Autodesk Inventor part; units mm, degrees
ref_plane "YZ Plane" through (0, 0, 0) normal (1, 0, 0) x (0, 1, 0)
ref_plane "XZ Plane" through (0, 0, 0) normal (0, 1, 0) x (-1, 0, 0)
ref_plane "XY Plane" through (0, 0, 0) normal (0, 0, 1) x (1, 0, 0)
sketch "Sketch1" plane through (0, 0, 0) normal (0, 0, 1) x (1, 0, 0)
  line L0 (-41, -50) -> (41, -50)
  line L1 (41, -50) -> (41, 50)
  line L2 (41, 50) -> (-41, 50)
  line L3 (-41, 50) -> (-41, -50)
  line L4 (-41, -50) -> (41, 50) construction
  line L5 (41, -50) -> (-41, 50) construction
  point P0 (0, 0)
  dimension "d154" = 82
  dimension "d155" = 100
extrude "Plate5" add sketch "Sketch1" along normal blind 2
sketch "Sketch7" plane through (-39, -50, 0) normal (-1, 0, 0) x (0, -1, 0)
  line L0 (-100, 0) -> (0, 0)
  line L1 (0, 0) -> (0, 84)
  line L2 (0, 84) -> (-100, 84)
  line L3 (-100, 84) -> (-100, 0)
edge flange "Flange3" height 84 angle 90 thickness 2 bend radius 2.75 thickness toward (-1, 0, 0) relief round relief width 2 relief depth 1 edges at (-41, 0, 2) wall of the first edge with corners at (-39, 50, 0) (-39, -50, 0) (-39, -50, 84) (-39, 50, 84)
bend "Bend3"
corner "Corner3"
sketch "Sketch8" plane through (0, 0, 2) normal (0, 0, 1) x (1, 0, 0)
  line L0 (41, 50) -> (41, -50)
  line L1 (-36.25, 50) -> (41, 50)
  line L2 (30.375, 42) -> (-25.625, 42)
  line L3 (-25.625, 42) -> (-25.625, -14)
  line L4 (-25.625, -14) -> (30.375, -14)
  line L5 (30.375, -14) -> (30.375, 42)
  line L6 (30.375, 42) -> (-25.625, -14) construction
  line L7 (-25.625, 42) -> (30.375, -14) construction
  point P0 (0, 0)
  point P1 (2.375, 14)
  point P2 (2.375, 50)
  dimension "d167" = 56
  dimension "d168" = 56
  dimension "d169" = 8
extrude "Cut1" cut sketch "Sketch8" against normal blind 2
sketch "Sketch9" plane through (-41, -50, 84) normal (-1, 0, 0) x (0, 0, 1)
  line L0 (-24.375, 44.75) -> (-54.875, 44.75)
  line L1 (-54.875, 44.75) -> (-54.875, 75.25)
  line L2 (-54.875, 75.25) -> (-24.375, 75.25)
  line L3 (-24.375, 75.25) -> (-24.375, 44.75)
  line L4 (-24.375, 44.75) -> (-54.875, 75.25) construction
  line L5 (-54.875, 44.75) -> (-24.375, 75.25) construction
  circle A0 centre (-16.625, 37) radius 2.5
  circle A1 centre (-62.625, 37) radius 2.5
  circle A2 centre (-62.625, 83) radius 2.5
  circle A3 centre (-16.625, 83) radius 2.5
  circle A4 centre (-39.625, 60) radius 32.5269 construction
  line L6 (-54.875, 44.75) -> (-62.625, 37) construction
  line L7 (-14.125, 34.5) -> (-65.125, 34.5) construction
  line L8 (-65.125, 34.5) -> (-65.125, 85.5) construction
  line L9 (-65.125, 85.5) -> (-14.125, 85.5) construction
  line L10 (-14.125, 85.5) -> (-14.125, 34.5) construction
  line L11 (-14.125, 34.5) -> (-65.125, 85.5) construction
  line L12 (-65.125, 34.5) -> (-14.125, 85.5) construction
  line L13 (-79.25, 100) -> (0, 100)
  line L14 (-39.625, 100) -> (-39.625, 60) construction
  circle A5 centre (-62.625, 83) radius 10.9602 construction
  line L15 (-16.625, 37) -> (-62.625, 37) construction
  line L16 (-62.625, 37) -> (-62.625, 83) construction
  line L17 (-62.625, 83) -> (-16.625, 83) construction
  line L18 (-16.625, 83) -> (-16.625, 37) construction
  line L19 (-16.625, 37) -> (-62.625, 83) construction
  line L20 (-62.625, 37) -> (-16.625, 83) construction
  point P0 (-84, 50)
  point P1 (-104.8197, 150.8767)
  point P2 (-104.8197, 150.8767)
  dimension "d181" = 21.9203
  dimension "d174" = 30.5
  dimension "d175" = 30.5
  dimension "d176" = 5
  dimension "d179" = 40
  dimension "d180" = 51
  dimension "d184" = 46
extrude "Cut2" cut sketch "Sketch9" against normal blind 2
properties part number "PRS 940-510 FDS Central tube wall" material "Stainless Steel"
Part model, mm, in its own coordinate system. A direction names the side the tool comes from. Coordinates: 2 decimals unless noted, no trailing zeros. Loops run counter-clockwise (first coordinate to the right, second up) from the corner with the lowest first, then second, coordinate; pieces in that order, holes last. Notation, with made-up numbers: (-1.75, 4.5) -> (46.25, 4.5) arc R17 cw to (46.25, 25.5) -> close; hole circle Ø2 at (3, 29.25). An arc over 180 degrees is marked (long way). Use a Markdown table: item, result. Add a question column.
Item 1: Band-saw the part on A-A on x = -21.5. Write the cut outline in (y, z), plus the area to 3 significant figures.
Item 2: Pull direction Y, two halves, no side cores. Call faces 1 (the flat face through (2, -22, 2)), 2 (the flat face through (-40, -50, 24)), 3 (the cylindrical face through (-40.014, 34.69, 19.532)): +Y half, -Y half, draft (parallel to the pull), parting line (faces both ways), or undercut.
Item 3: Band-saw the part on D-D on y = 3.5. Write the cut outline in (x, z) (3 decimals), plus the area to 3 significant figures.
Item 4: Probe probe 1 along X at (y, z) = (25, 60); probe 2 along Z at (x, y) = (28, -29). List the from-to ranges inside material, lowest first.
Item 5: Band-saw the part on B-B on y = 33. Write the cut outline in (x, z) (3 decimals).
Item 6: Band-saw the part on C-C on y = -40.5. Write the cut outline in (x, z), plus the area to 3 significant figures.
Item 7: Which spindle directions (+Z, -Z, +X, -X, +Y, -Y) get a long thin tool onto all of the face, cutting with end or side? Do faces 4 (the cylindrical face through (-40.01, -14.52, 19.39)), 5 (the flat face through (-39, -12, 44)). Say none if no direction does.
Item 8: Flat gauge pins, fed straight in: P1, Ø0.6, axis at y = 3.5, z = 0.5, coming from the -X side; P2, Ø24, axis at y = -23, z = 54.5, coming from the +X side; P3, Ø2, axis at x = -40.5, y = 12, coming from the -Z side. Where does each tip first touch, or does it go through?
Geometry says:
| question | item | result |
|---|---|---|
| 1 | outline | (-50, 0) -> (-14, 0) -> (-14, 2) -> (-50, 2) -> close; (42, 0) -> (50, 0) -> (50, 2) -> (42, 2) -> close |
| 1 | area | 88.0 mm² |
| 2 | face 1 | draft |
| 2 | face 2 | -Y half |
| 2 | face 3 | undercut |
| 3 | outline | (-41, 4.75) arc R4.75 ccw to (-36.25, 0) -> (-25.625, 0) -> (-25.625, 2) -> (-36.25, 2) arc R2.75 cw to (-39, 4.75) -> (-39, 29.125) -> (-41, 29.125) -> close; (-41, 59.625) -> (-39, 59.625) -> (-39, 84) -> (-41, 84) -> close; (30.375, 0) -> (41, 0) -> (41, 2) -> (30.375, 2) -> close |
| 3 | area | 152 mm² |
| 4 | probe 1 | -41 to -39 |
| 4 | probe 2 | 0 to 2 |
| 5 | outline | (-41, 4.75) arc R4.75 ccw to (-36.25, 0) -> (-25.625, 0) -> (-25.625, 2) -> (-36.25, 2) arc R2.75 cw to (-39, 4.75) -> (-39, 18.875) -> (-41, 18.875) -> close; (-41, 23.875) -> (-39, 23.875) -> (-39, 64.875) -> (-41, 64.875) -> close; (-41, 69.875) -> (-39, 69.875) -> (-39, 84) -> (-41, 84) -> close; (30.375, 0) -> (41, 0) -> (41, 2) -> (30.375, 2) -> close |
| 6 | outline | (-41, 4.75) arc R4.75 ccw to (-36.25, 0) -> (41, 0) -> (41, 2) -> (-36.25, 2) arc R2.75 cw to (-39, 4.75) -> (-39, 84) -> (-41, 84) -> close |
| 6 | area | 325 mm² |
| 7 | face 4 | +X, -X |
| 7 | face 5 | +Z, +X, +Y, -Y |
| 8 | P1 | x = -38.89 |
| 8 | P2 | x = -39 |
| 8 | P3 | z = 1.29 |
